Model file for the job. Use its own axes, mm. A direction names the side the tool comes from. Round coordinates to 2 decimals unless told otherwise and drop trailing zeros. Loops run counter-clockwise (first coordinate to the right, second up) from the corner with the lowest first, then second, coordinate; pieces in that order, holes last. Notation, with made-up numbers: (45, 76) -> (73, 76) arc R13 ccw to (73, 93) -> close; hole circle Ø1 at (66, 65.25). An arc over 180 degrees is marked (long way). Use a Markdown table: item, result. Add a question column.
Autodesk Inventor part; units mm, degrees
ref_plane "YZ Plane" through (0, 0, 0) normal (1, 0, 0) x (0, 1, 0)
ref_plane "XZ Plane" through (0, 0, 0) normal (0, 1, 0) x (-1, 0, 0)
ref_plane "XY Plane" through (0, 0, 0) normal (0, 0, 1) x (1, 0, 0)
sketch "Boceto1" plane through (0, 0, 0) normal (1, 0, 0) x (0, 1, 0)
  circle A0 centre (0, 0) radius 5.9
  dimension "d0" = 11.8
extrude "Extrusión1" add sketch "Boceto1" along normal blind 3
sketch "Boceto2" plane through (3, 0, 0) normal (1, 0, 0) x (0, 0, -1)
  circle A0 centre (0, 0) radius 7.5
  dimension "d3" = 15
extrude "Extrusión2" add sketch "Boceto2" against normal blind 1.5
sketch "Boceto3" plane through (0, 0, 0) normal (-1, 0, 0) x (0, 0, 1)
  circle A0 centre (0, 0) radius 4.75
  dimension "d6" = 9.5
extrude "Extrusión3" cut sketch "Boceto3" against normal blind 2
fillet "Empalme1" radius 1 1 edges at (3, 0, 7.5)
sketch "Boceto4" plane through (3, 0, 0) normal (1, 0, 0) x (0, 0, -1)
  circle A0 centre (0, 0) radius 0.6
  dimension "d13" = 1.2
extrude "Extrusión4" cut sketch "Boceto4" against normal blind 10
sketch "Boceto5" plane through (0, 0, 0) normal (-1, 0, 0) x (0, 0, 1)
  circle A0 centre (0, 0) radius 5.9
  circle A1 centre (0, 0) radius 5.9
  circle A2 centre (0, 0) radius 4.75
extrude "Extrusión5" add sketch "Boceto5" along normal blind 1.5
chamfer "Chaflán2" distance 1 angle 45 1 edges at (-1.5, 0, -5.9)
properties part number "tapa carcasa camara"
1) Wall check: probe 1 along X at (y, z) = (1.5, 4.25); probe 2 along Y at (x, z) = (2.5, 0); probe 3 along Z at (x, y) = (1.75, -3.25). Give the ranges that are in metal, low to high. Write a range as from..to.
2) Pull direction Z, two halves, no side cores. Call faces 1 (the face through (0.514, 5.476, 2.196)), 2 (the face through (1.5, -2, 6)), 3 (the face through (0.274, 4.214, 2.192)): +Z half, -Z half, draft (parallel to the pull), parting line (faces both ways), or undercut.
3) Cut at A-A on x = -1.2. Write the cut outline in (y, z), and give its area (3 significant figures).
4) Tool access for faces 4 (the face through (3, 0, -1)), 5 (the face through (2, -1, 0)): list every direction of +Z, -Z, +X, -X, +Y, -Y with a clear straight run to the whole face (end or side of a thin tool).
5) Cut at B-B on x = 0.7. Write the cut outline in (y, z), and give its area (3 significant figures).
6) Pin check, flat tips, straight feed: pin 1 Ø1.5 at (x, y) = (0.5, 4.5) entering from +Z; pin 2 Ø2 at (x, z) = (0, 4.5) entering from +Y. Stop position of each tip, or through.
Established:
| question | item | result |
|---|---|---|
| 1 | probe 1 | x = 2..3 |
| 1 | probe 2 | y = -7.37..-0.6, 0.6..7.37 |
| 1 | probe 3 | z = -6.76..-3.46, 3.46..6.76 |
| 2 | face 1 | parting line |
| 2 | face 2 | draft |
| 2 | face 3 | undercut |
| 3 | outline | circle Ø10.4 at (0, 0); hole circle Ø9.5 at (0, 0) |
| 3 | area | 14.1 mm^2 |
| 4 | face 4 | +Z, -Z, +X, +Y, -Y |
| 4 | face 5 | -X |
| 5 | outline | circle Ø11.8 at (0, 0); hole circle Ø9.5 at (0, 0) |
| 5 | area | 38.5 mm^2 |
| 6 | pin 1 | stops at z = 4.55 |
| 6 | pin 2 | stops at y = 4.75 |
